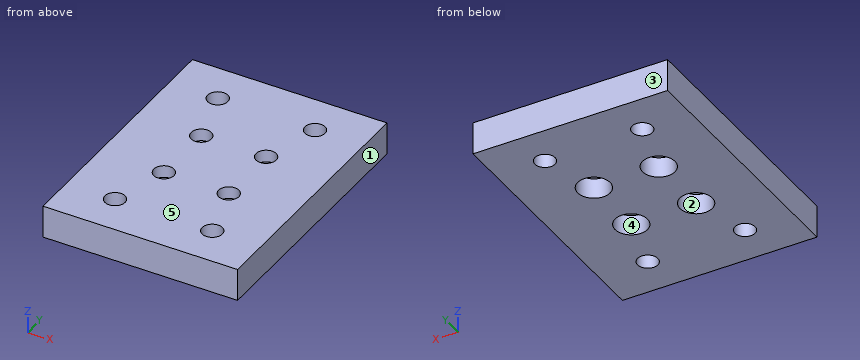
Autodesk Inventor part; units mm, degrees
ref_plane "YZ Plane" through (0, 0, 0) normal (1, 0, 0) x (0, 1, 0)
ref_plane "XZ Plane" through (0, 0, 0) normal (0, 1, 0) x (-1, 0, 0)
ref_plane "XY Plane" through (0, 0, 0) normal (0, 0, 1) x (1, 0, 0)
sketch "Sketch1" plane through (0, 0, 0) normal (0, 0, 1) x (1, 0, 0)
  line L0 (246.3741, 31.7234) -> (246.3741, -882.6766) construction
  line L1 (234.1821, 31.7234) -> (231.3881, 31.7234) construction
  line L2 (223.2601, 31.7234) -> (220.4661, 31.7234) construction
  line L3 (199.5111, 31.7234) -> (196.0821, 31.7234) construction
  line L4 (182.3661, 31.7234) -> (178.9371, 31.7234) construction
  line L5 (246.3741, 31.7234) -> (170.1741, 31.7234)
  line L6 (170.1741, 31.7234) -> (170.1741, -69.8766)
  line L7 (170.1741, -69.8766) -> (246.3741, -69.8766)
  line L8 (246.3741, -69.8766) -> (246.3741, 31.7234)
  circle A0 centre (227.3241, 15.8484) radius 3.9688
  line L9 (208.2741, -69.8766) -> (208.2741, 31.7234) construction
  line L10 (246.3741, -19.0766) -> (170.1741, -19.0766) construction
  circle A1 centre (227.3241, -54.0016) radius 3.9688
  circle A2 centre (189.2241, 15.8484) radius 3.9688
  circle A3 centre (189.2241, -54.0016) radius 3.9688
  point P0 (0, 0)
  dimension "d0" = 76.2
  dimension "d1" = 101.6
  dimension "d2" = 7.9375
  dimension "d3" = 15.875
  dimension "d4" = 19.05
extrude "Extrusion1" add sketch "Sketch1" along normal blind 12.7
sketch "Sketch3" plane through (0, 0, 0) normal (0, 0, -1) x (-1, 0, 0)
  line L0 (-186.0491, -41.3016) -> (-230.4991, -41.3016)
  line L1 (-230.4991, -41.3016) -> (-230.4991, 3.1484)
  line L2 (-230.4991, 3.1484) -> (-186.0491, 3.1484)
  line L3 (-186.0491, 3.1484) -> (-186.0491, -41.3016)
  line L4 (-170.1741, -69.8766) -> (-246.3741, -69.8766)
  line L5 (-170.1741, 31.7234) -> (-170.1741, -69.8766)
  line L6 (-246.3741, 31.7234) -> (-170.1741, 31.7234)
  circle A0 centre (-195.5741, -6.3766) radius 6.35
  circle A1 centre (-195.5741, -31.7766) radius 6.35
  circle A2 centre (-220.9741, -6.3766) radius 6.35
  circle A3 centre (-220.9741, -31.7766) radius 6.35
  point P0 (0, 0)
  dimension "d16" = 44.45
  dimension "d17" = 44.45
  dimension "d18" = 28.575
  dimension "d19" = 15.875
  dimension "d23" = 12.7
  dimension "d24" = 9.525
  dimension "d25" = 9.525
  dimension "d28" = 25.4
  dimension "d31" = 25.4
extrude "Extrusion3" cut sketch "Sketch3" against normal blind 7.9375 contours A0 | A1 | A2 | A3
sketch "Sketch4" plane through (195.5741, -6.3766, 7.9375) normal (0, 0, -1) x (-1, 0, 0)
  circle A0 centre (0, 0) radius 6.35
  circle A1 centre (0, -25.4) radius 6.35
  circle A2 centre (-25.4, 0) radius 6.35
  circle A3 centre (-25.4, -25.4) radius 6.35
  circle A4 centre (0, 0) radius 3.9688
  line L0 (0, 0) -> (0, -11.1628) construction
  line L1 (0, 0) -> (-15.7699, 0) construction
  circle A5 centre (0, -25.4) radius 3.9688
  circle A6 centre (-25.4, 0) radius 3.9688
  circle A7 centre (-25.4, -25.4) radius 3.9688
  point P0 (195.5741, 6.3766)
  dimension "d36" = 7.9375
  dimension "d37" = 7.9375
  dimension "d38" = 7.9375
  dimension "d39" = 7.9375
extrude "Extrusion4" cut sketch "Sketch4" against normal blind 7.9375 contours A4 | A5 | A6 | A7
properties part number "Corner Stands"
CAD build for the part. Positions are in the model's coordinates, mm. Face numbers are marked on the shaded views. A direction names the side the tool comes from. Round coordinates to 2 decimals unless told otherwise and drop trailing zeros. Order: outer loops, then holes, each group sorted by start corner. A loop starts at its lowest first (then second) coordinate and runs counter-clockwise, first axis right, second up. Notation, with made-up numbers: M -17.5,23.5 L 30.5,23.5 A28 cw 30.5,61.5 Z; hole C 82,27 d6. An arc over 180 degrees is marked long. Use one line per item in the form item = value.
Q1. Probe L1, parallel to Y at x = 220, z = 10.25; L2, parallel to Y at x = 222.5, z = 9.75; L3, parallel to Y at x = 226, z = 7.75. List the from-to ranges inside material, lowest first.
Recorded:
L1 = -69.88 to -35.62, -27.93 to -10.22, -2.53 to 31.72
L2 = -69.88 to -35.44, -28.11 to -10.04, -2.71 to 31.72
L3 = -69.88 to -57.74, -50.26 to -35.66, -27.9 to -10.26, -2.5 to 12.11, 19.59 to 31.72
Q2. Two-plate mould, pull along Y, no slides. Class the marked faces 3, 4 and 5: +Y half, -Y half, draft (parallel to the pull), parting line (faces both ways), or undercut.
Recorded:
face_3 = +Y half
face_4 = undercut
face_5 = draft
Q3. Flat gauge pins, fed straight in: P1, Ø10, axis at x = 220.97, y = -6.38, coming from the -Z side; P2, Ø5, axis at x = 189.22, y = -54, coming from the +Z side. Where does each tip first touch, or does it go through?
Recorded:
P1 = 7.94
P2 = through
Q4. Saw through at B-B on z = 11.5. State how many separate pieces and enclosed holes the cut face has, then the cut area to 3 significant figures.
Recorded:
separate_pieces = 1
enclosed_holes = 8
area = 7,350 mm^2
Q5. Saw through at A-A on y = -52. Give the cut face in (x, z).
Recorded:
outline = M 170.17,0 L 185.8,0 L 185.8,12.7 L 170.17,12.7 Z; M 192.65,0 L 223.9,0 L 223.9,12.7 L 192.65,12.7 Z; M 230.75,0 L 246.37,0 L 246.37,12.7 L 230.75,12.7 Z
Q6. Which spindle directions (+Z, -Z, +X, -X, +Y, -Y) get a long thin tool onto all of the face, cutting with end or side? Do the marked faces 1 and 2. Say none if no direction does.
Recorded:
face_1 = +Z, -Z, +X, +Y, -Y
face_2 = -Z
Q7. Saw through at C-C on x = 221.5. Give the cut face in (y, z).
Recorded:
outline = M -69.88,0 L -38.1,0 L -38.1,7.94 L -35.71,7.94 L -35.71,12.7 L -69.88,12.7 Z; M -27.84,7.94 L -25.45,7.94 L -25.45,0 L -12.7,0 L -12.7,7.94 L -10.31,7.94 L -10.31,12.7 L -27.84,12.7 Z; M -2.44,7.94 L -0.05,7.94 L -0.05,0 L 31.72,0 L 31.72,12.7 L -2.44,12.7 Z
Q8. Saw through at D-D on y = 14.5. Give the cut face in (x, z), then the cut area to 3 significant figures.
Recorded:
outline = M 170.17,0 L 185.49,0 L 185.49,12.7 L 170.17,12.7 Z; M 192.96,0 L 223.59,0 L 223.59,12.7 L 192.96,12.7 Z; M 231.06,0 L 246.37,0 L 246.37,12.7 L 231.06,12.7 Z
area = 778 mm^2
